Work out the finished part from the listing and answer in its coordinate system (mm). A direction names the side the tool comes from. Coordinates: 2 decimals unless noted, no trailing zeros. Write each loop counter-clockwise with the first axis right and the second up, starting at its lowest first coordinate (ties: lowest second). Pieces come first, ordered by that corner, then holes. Notation, with made-up numbers: (-22.75, -9.5) - (-4.75, -9.5) arc R23 ccw to (-4.75, 2.5) - close; hole circle Ø7 at (32, 14.25). An arc over 180 degrees is marked (long way). Use a Markdown table: item, result. Add a question column.
(1) The part is cut by section A-A, the plane y = -85. Give the vertices of the cut face in (x, z), then the cut area to 3 significant figures.
(2) A tool of negligible diameter and unlimited length cuts with its end or side. For faces 4 (the face through (97, 0, -133)), 5 (the face through (158.793, -114.833, 1.954)), 6 (the face through (100, -13, -101.6)), from which of +Z, -Z, +X, -X, +Y, -Y can it reach the whole face along a straight path? Write none if from no direction.
(3) The part is cut by section D-D, the plane z = 0. State how many separate pieces and enclosed holes the cut face has, then the cut area to 3 significant figures.
(4) The part is cut by section B-B, the plane y = -9.5. Give the vertices of the cut face in (x, z).
(5) For a pull along Z with two mould halves and no side action, classify faces 1 (the face through (406.35, -37.57, -4.47)), 2 (the face through (100, -114, -127)), 3 (the face through (103, -13, 101.6)) as released by +Z, released by -Z, zero draft, split by the parting line, or undercut.
(6) The part is cut by section C-C, the plane x = 71. Give the vertices of the cut face in (y, z), then the cut area to 3 significant figures.
(7) Given pin 1 Ø3 at (x, z) = (-114, -150) entering from -Y; pin 2 Ø1 at (y, z) = (-20, 39) entering from +X; pin 3 Ø2 at (y, z) = (-45, -67.5) entering from +X, each flat-ended and moving along its own axis, determine where each tip first touches the part or whether it passes through.
(8) Find the intervals of material crossed by line 1 (Z direction, x = 203.2, y = -108.5); line 2 (Z direction, x = 110, y = -122); line 3 (Y direction, x = 223, z = 41.5), in increasing order. Write a range as from..to.
from build123d import *

# Parameters (mm, degrees)
F1_DEPTH       = 76.2
F2_DEPTH       = 152.4
F3_R           = 44.45
F4_DEPTH       = 76.2
F6_D           = 25.4
F6_CSINK_D     = 50.8
F6_CSINK_ANGLE = 90
F8_DEPTH       = 25.4


with BuildPart() as f1:
    # F0 (on Front) → F1 (new body)
    with BuildSketch(Plane.XZ):
        with BuildLine():
            Line((203.2, 203.2), (0, 203.2))
            ThreePointArc((0, 203.2), (-203.2, 0), (0, -203.2))
            Line((0, -203.2), (203.2, -203.2))
            ThreePointArc((203.2, -203.2), (406.4, 0), (203.2, 203.2))
        make_face()
        with BuildLine():
            ThreePointArc((0, -127), (-127, 0), (0, 127))
            Line((0, 127), (203.2, 127))
            ThreePointArc((203.2, 127), (330.2, 0), (203.2, -127))
            Line((203.2, -127), (0, -127))
        make_face(mode=Mode.SUBTRACT)
        with BuildLine():
            Line((203.2, 127), (0, 127))
            ThreePointArc((0, 127), (-127, 0), (0, -127))
            Line((0, -127), (203.2, -127))
            ThreePointArc((203.2, -127), (330.2, 0), (203.2, 127))
        make_face()
    extrude(amount=F1_DEPTH)

    # F0 (on Front) → F2 (join)
    with BuildSketch(Plane.XZ):
        with BuildLine():
            Line((203.2, 127), (0, 127))
            ThreePointArc((0, 127), (-127, 0), (0, -127))
            Line((0, -127), (203.2, -127))
            ThreePointArc((203.2, -127), (330.2, 0), (203.2, 127))
        make_face()
    extrude(amount=F2_DEPTH)

    # F3 (on face) → F4 (cut)
    with BuildSketch(Plane.XZ.offset(152.4)):
        with BuildLine():
            Line((203.2, 76.2), (0, 76.2))
            ThreePointArc((0, 76.2), (-76.2, 0), (0, -76.2))
            Line((0, -76.2), (203.2, -76.2))
            ThreePointArc((203.2, -76.2), (279.4, 0), (203.2, 76.2))
        make_face()
        Circle(F3_R, mode=Mode.SUBTRACT)
        with Locations((203.2, 0)):
            Circle(F3_R, mode=Mode.SUBTRACT)
    extrude(amount=-F4_DEPTH, mode=Mode.SUBTRACT)

    # F6 (through all)
    with Locations(Plane.XZ.offset(152.4)):
        with Locations((0, 0), (203.2, 0)):
            CounterSinkHole(F6_D / 2, F6_CSINK_D / 2, counter_sink_angle=F6_CSINK_ANGLE)

    # F7 (on face) → F8 (cut)
    with BuildSketch(Plane.XZ):
        with BuildLine():
            Line((203.2, 101.6), (0, 101.6))
            ThreePointArc((0, 101.6), (-101.6, 0), (0, -101.6))
            Line((0, -101.6), (203.2, -101.6))
            ThreePointArc((203.2, -101.6), (304.8, 0), (203.2, 101.6))
        make_face()
    extrude(amount=F8_DEPTH, mode=Mode.SUBTRACT)


solid = f1.part
Model answer:
| question | item | result |
|---|---|---|
| 1 | outline | circle Ø88.9 at (0, 0); (0, -127) - (203.2, -127) arc R127 ccw to (203.2, 127) - (0, 127) arc R127 ccw to start; circle Ø88.9 at (203.2, 0); hole circle Ø25.4 at (0, 0); hole (0, -76.2) - (203.2, -76.2) arc R76.2 ccw to (203.2, 76.2) - (0, 76.2) arc R76.2 ccw to start; hole circle Ø25.4 at (203.2, 0) |
| 1 | area | 64,500 mm^2 |
| 2 | face 4 | +Z, -Z, +X, -X, +Y |
| 2 | face 5 | -Y |
| 2 | face 6 | +Y |
| 3 | separate pieces | 3 |
| 3 | enclosed holes | 0 |
| 3 | area | 50,600 mm^2 |
| 4 | outline | (0, -203.2) - (203.2, -203.2) arc R203.2 ccw to (203.2, 203.2) - (0, 203.2) arc R203.2 ccw to start; hole (0, -101.6) - (203.2, -101.6) arc R101.6 ccw to (203.2, 101.6) - (0, 101.6) arc R101.6 ccw to start |
| 5 | face 1 | split by the parting line |
| 5 | face 2 | released by -Z |
| 5 | face 3 | undercut |
| 6 | outline | (-152.4, -127) - (-76.2, -127) - (-76.2, -203.2) - (0, -203.2) - (0, -101.6) - (-25.4, -101.6) - (-25.4, 101.6) - (0, 101.6) - (0, 203.2) - (-76.2, 203.2) - (-76.2, 127) - (-152.4, 127) - (-152.4, 76.2) - (-76.2, 76.2) - (-76.2, -76.2) - (-152.4, -76.2) - close |
| 6 | area | 33,500 mm^2 |
| 7 | pin 1 | y = -76.2 |
| 7 | pin 2 | x = 402.72 |
| 7 | pin 3 | x = 395.21 |
| 8 | line 1 | -127..-76.2, -44.45..-12.7, 12.7..44.45, 76.2..127 |
| 8 | line 2 | -127..-76.2, 76.2..127 |
| 8 | line 3 | -76.2..-25.4 |
